```python
from build123d import *

# Parameters (mm, degrees)
F0_W          = 76.2
F0_H          = 127
F0_W_2        = 63.5
F0_H_2        = 114.3
F1_DEPTH      = 914.4
F2_R          = 19.05
F3_DEPTH      = 127.001
F5_DEPTH      = 63.5
F5_DEPTH_BACK = 63.5
F7_DEPTH      = 63.5
F7_DEPTH_BACK = 63.5
F9_DEPTH      = 63.5
F9_DEPTH_BACK = 63.5


with BuildPart() as f1:
    # F0 (on Front) → F1 (new body, symmetric)
    with BuildSketch(Plane.XZ):
        with Locations((-38.1, 0)):
            Rectangle(F0_W, F0_H)
        with Locations((-38.1, 0)):
            Rectangle(F0_W_2, F0_H_2, mode=Mode.SUBTRACT)
    extrude(amount=F1_DEPTH, both=True)

    # F2 (on face) → F3 (cut, through all)
    with BuildSketch(Plane.XY.offset(63.5)):
        with Locations((-38.1, 787.4)):
            Circle(F2_R)
    extrude(amount=-F3_DEPTH, mode=Mode.SUBTRACT)

    # F4 (on Top) → F5 (cut, two sides)
    with BuildSketch(Plane.XY) as f5_sk:
        Polygon((0, -863.6), (-50.8, -914.4), (0, -914.4), align=None)
        Polygon((0, 863.6), (0, 914.4), (-50.8, 914.4), align=None)
    extrude(amount=F5_DEPTH, mode=Mode.SUBTRACT)
    extrude(f5_sk.sketch, amount=-F5_DEPTH_BACK, mode=Mode.SUBTRACT)

    # F6 (on Top) → F7 (join, two sides)
    with BuildSketch(Plane.XY) as f7_sk:
        Polygon((-76.2, -908.05), (-76.2, -914.4), (-50.8, -914.4), (0, -863.6), (0, -854.619744), (-53.430256, -908.05), align=None)
    extrude(amount=F7_DEPTH)
    extrude(f7_sk.sketch, amount=-F7_DEPTH_BACK)

    # F8 (on Top) → F9 (join, two sides)
    with BuildSketch(Plane.XY) as f9_sk:
        Polygon((-50.8, 914.4), (-76.2, 914.4), (-76.2, 908.05), (-53.430256, 908.05), (0, 854.619744), (0, 863.6), align=None)
    extrude(amount=F9_DEPTH)
    extrude(f9_sk.sketch, amount=-F9_DEPTH_BACK)


solid = f1.part
```
Here's how the part is built. I have some questions about the finished solid (model axes, mm). A direction names the side the tool comes from. Round coordinates to 2 decimals unless told otherwise and drop trailing zeros. Write each loop counter-clockwise with the first axis right and the second up, starting at its lowest first coordinate (ties: lowest second). Pieces come first, ordered by that corner, then holes.
Q1. If we mould it in two halves opening along Y, with no side actions, what happens to faces 1 (the flat face through (-25, 888.6, 0.9)), 2 (the flat face through (-6.35, -12, -1)), 3 (the flat face through (-39, -13, 63.5)), 4 (the flat face through (-29.56, -884.18, -0.8))? For each: +Y half, -Y half, draft (parallel to the pull), parting line (faces both ways), or undercut.
Q2. If we section it at C-C on y = 177: Write out the boundary of the cut face in (x, z).
Q3. If we section it at A-A on y = 787.4: Write out the boundary of the cut face in (x, z), plus the area to 3 significant figures.
Q4. Will these pins go through, and if not, where does the flat tip stop? P1, Ø1.5, axis at x = -9, z = 33, coming from the +Y side; P2, Ø2, axis at x = -27.5, z = -14.5, coming from the -Y side.
Q5. Please list where these lines run through material, in increasing order: probe 1 along X at (y, z) = (-307.5, -13); probe 2 along Z at (x, y) = (-43, 281); probe 3 along Y at (x, z) = (-66.5, 21).
Q6. Which directions (+Z, -Z, +X, -X, +Y, -Y) give clear straight access to the entire face, cutting with the end or side of a thin tool? Please do faces 5 (the flat face through (-76.2, -13, -1)), 6 (the flat face through (-39, -13, -57.15)).
Q7. If we section it at D-D on x = -38.1: Write out the boundary of the cut face in (y, z), plus the area to 3 significant figures.
Q8. If we section it at B-B on z = -7.5: Write out the boundary of the cut face in (x, y), plus the area to 3 significant figures.
Answer below:
1. face 1: +Y half
1. face 2: undercut
1. face 3: draft
1. face 4: undercut
2. outline: (-76.2, -63.5) - (0, -63.5) - (0, 63.5) - (-76.2, 63.5) - close; hole (-69.85, -57.15) - (-6.35, -57.15) - (-6.35, 57.15) - (-69.85, 57.15) - close
3. outline: (-76.2, -63.5) - (-57.15, -63.5) - (-57.15, -57.15) - (-69.85, -57.15) - (-69.85, 57.15) - (-57.15, 57.15) - (-57.15, 63.5) - (-76.2, 63.5) - close; (-19.05, -63.5) - (0, -63.5) - (0, 63.5) - (-19.05, 63.5) - (-19.05, 57.15) - (-6.35, 57.15) - (-6.35, -57.15) - (-19.05, -57.15) - close
3. area: 1,940 mm2
4. P1: stops at y = 873.35
4. P2: stops at y = -892.1
5. probe 1: x = -76.2 to -69.85, -6.35 to 0
5. probe 2: z = -63.5 to -57.15, 57.15 to 63.5
5. probe 3: y = -914.4 to -908.05, 908.05 to 914.4
6. face 5: +Z, -Z, -X, +Y, -Y
6. face 6: none
7. outline: (-901.7, -63.5) - (768.35, -63.5) - (768.35, -57.15) - (-892.72, -57.15) - (-892.72, 57.15) - (768.35, 57.15) - (768.35, 63.5) - (-901.7, 63.5) - close; (806.45, -63.5) - (901.7, -63.5) - (901.7, 63.5) - (806.45, 63.5) - (806.45, 57.15) - (892.72, 57.15) - (892.72, -57.15) - (806.45, -57.15) - close
7. area: 24,500 mm2
8. outline: (-76.2, -914.4) - (-50.8, -914.4) - (0, -863.6) - (0, 863.6) - (-50.8, 914.4) - (-76.2, 914.4) - close; hole (-69.85, -908.05) - (-53.43, -908.05) - (-6.35, -860.97) - (-6.35, 860.97) - (-53.43, 908.05) - (-69.85, 908.05) - close
8. area: 23,700 mm2
